```python
from build123d import *

# Parameters (mm, degrees)
BASPROSKE_W        = 7
BASPROSKE_H        = 7
TOOTHCUT_DEPTH     = 13.124355653
TEETHCUTS_COUNT    = 12
TEETHCUTS_ANGLE    = 330
BORSKE_R           = 0.4
BORE_DEPTH         = 50.0000508
CUT_EXTRUDE1_DEPTH = 12.89949757
SKETCH2_R          = 8.839336396
CUT_EXTRUDE2_DEPTH = 1


with BuildPart() as part:
    # BasProSke → Base-Revolve (revolve)
    with BuildSketch(Plane(origin=(0, 0, 0), x_dir=(1, 0, 0), z_dir=(0, 1, 0)), mode=Mode.PRIVATE) as base_revolve_sk:
        with Locations((3.5, 3.5)):
            Rectangle(BASPROSKE_W, BASPROSKE_H)
    revolve(base_revolve_sk.sketch.rotate(Axis((-10, 0, 0), (1, 0, 0)), 180), axis=Axis((-10, 0, 0), (1, 0, 0)))

    # TooCutSke → ToothCut (cut, through all)
    with BuildSketch(Plane(origin=(0, 0, 0), x_dir=(0, 0, -1), z_dir=(1, 0, 0))):
        with BuildLine():
            ThreePointArc((0.562207301, 4.715604304), (0, 4.749), (-0.562207301, 4.715604304))
            ThreePointArc((-0.562207301, 4.715604304), (-0.837528627, 5.917009812), (-1.672850686, 6.823328788))
            ThreePointArc((-1.672850686, 6.823328788), (0, 7.0254), (1.672850686, 6.823328788))
            ThreePointArc((1.672850686, 6.823328788), (0.837528627, 5.917009812), (0.562207301, 4.715604304))
        make_face()
    toothcut = extrude(amount=TOOTHCUT_DEPTH, mode=Mode.SUBTRACT)

    # TeethCuts: ToothCut ×12 about axis
    teethcuts_axis = Axis((-10, 0, 0), (1, 0, 0))
    for i in range(1, TEETHCUTS_COUNT):
        add(toothcut.rotate(teethcuts_axis, i * TEETHCUTS_ANGLE / (TEETHCUTS_COUNT - 1)), mode=Mode.SUBTRACT)

    # BorSke → Bore (cut, symmetric)
    with BuildSketch(Plane(origin=(0, 0, 0), x_dir=(0, 0, -1), z_dir=(1, 0, 0))):
        with Locations(Location((0, 0, 0), (0, 0, 180))):
            Circle(BORSKE_R)
    extrude(amount=BORE_DEPTH, both=True, mode=Mode.SUBTRACT)

    # Sketch1 → Cut-Extrude1 (cut, through all)
    with BuildSketch(Plane(origin=(7, 0, 0), x_dir=(0, 0, -1), z_dir=(1, 0, 0))):
        with BuildLine():
            Line((-2.655654345, 1.5), (2.655654345, 1.5))
            ThreePointArc((2.655654345, 1.5), (0, -3.05), (-2.655654345, 1.5))
        make_face()
    extrude(amount=-CUT_EXTRUDE1_DEPTH, mode=Mode.SUBTRACT)

    # Sketch2 → Cut-Extrude2 (cut)
    with BuildSketch(Plane.ZY):
        Circle(SKETCH2_R)
    extrude(amount=-CUT_EXTRUDE2_DEPTH, mode=Mode.SUBTRACT)


solid = part.part
```
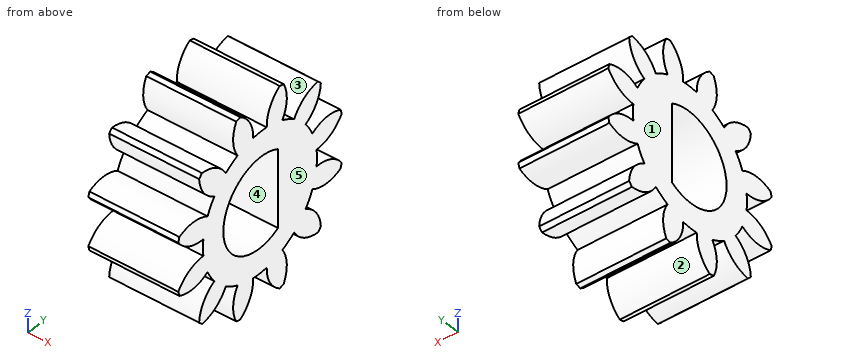
Design review of the part built by this model. Coordinates are the model's own, in mm. Face numbers are marked on the shaded views. A direction names the side the tool comes from. Coordinates: 2 decimals unless noted, no trailing zeros. Loops run counter-clockwise (first coordinate to the right, second up) from the corner with the lowest first, then second, coordinate; pieces in that order, holes last.
Q1. The part is to be moulded in two halves that separate along Y. For the marked faces 1, 2 and 3, say which applies: +Y half, -Y half, draft (parallel to the pull), parting line (faces both ways), or undercut.
Reported:
face 1: draft
face 2: undercut
face 3: undercut
Q2. Tool access review of the marked faces 4 and 5: name each direction out of +Z, -Z, +X, -X, +Y, -Y from which nothing blocks a thin tool from reaching the whole face with its end or side.
Reported:
face 4: +X, -X
face 5: +Z, -Z, +X, +Y, -Y
Q3. We need section A-A on y = 0. State the section outline as (x, z) points, and give its area (3 significant figures).
Reported:
outline: (1, -4.75) - (7, -4.75) - (7, -3.05) - (1, -3.05) - close; (1, 3.05) - (7, 3.05) - (7, 4.75) - (1, 4.75) - close
area: 20.4 mm2
Q4. We need section C-C on y = -4. State the section outline as (x, z) points, and give its area (3 significant figures).
Reported:
outline: (1, -4.87) - (7, -4.87) - (7, -2.96) - (1, -2.96) - close; (1, -2.56) - (7, -2.56) - (7, 2.56) - (1, 2.56) - close; (1, 2.96) - (7, 2.96) - (7, 4.87) - (1, 4.87) - close
area: 53.7 mm2
Q5. We need section B-B on z = 0. State the section outline as (x, y) points, and give its area (3 significant figures).
Reported:
outline: (1, -4.75) - (7, -4.75) - (7, -3.05) - (1, -3.05) - close; (1, 1.5) - (7, 1.5) - (7, 4.75) - (1, 4.75) - close
area: 29.7 mm2
Q6. To check wall thickness, follow line 1 (Z direction, x = 5.2, y = -4); line 2 (Z direction, x = 1.55, y = -0.75); line 3 (Y direction, x = 1.5, z = -1). State the ranges of each line that lie inside material, in increasing order.
Reported:
line 1: z = -4.87 to -2.96, -2.56 to 2.56, 2.96 to 4.87
line 2: z = -5.73 to -2.96, 2.96 to 5.73
line 3: y = -6.18 to -2.88, 1.5 to 6.18
